```python
from build123d import *

# Parameters (mm, degrees)
SKETCH1_R           = 11
BOSS_EXTRUDE2_DEPTH = 8
SKETCH3_R           = 3
SKETCH3_R_2         = 1.5
CUT_EXTRUDE2_DEPTH  = 12
CUT_EXTRUDE3_START  = -4
SKETCH4_R           = 11
SKETCH4_R_2         = 4.5
CUT_EXTRUDE3_DEPTH  = 4
SKETCH6_R           = 3.5
CUT_EXTRUDE4_DEPTH  = 10


with BuildPart() as part:
    # Sketch1 → Boss-Extrude2 (new body)
    with BuildSketch(Plane(origin=(0, 0, 0), x_dir=(1, 0, 0), z_dir=(0, 1, 0))):
        with Locations(Location((0, 0, 0), (0, 0, 270))):
            Circle(SKETCH1_R)
    extrude(amount=BOSS_EXTRUDE2_DEPTH)

    # Sketch3 → Cut-Extrude2 (cut)
    with BuildSketch(Plane(origin=(0, 8, 0), x_dir=(1, 0, 0), z_dir=(0, 1, 0))):
        with Locations(Location((0, 0, 0), (0, 0, 270))):
            Circle(SKETCH3_R)
        with Locations(Location((-7, 0, 0), (0, 0, 270))):
            Circle(SKETCH3_R_2)
        with Locations(Location((0, 7, 0), (0, 0, 270))):
            Circle(SKETCH3_R_2)
        with Locations(Location((7, 0, 0), (0, 0, 270))):
            Circle(SKETCH3_R_2)
        with Locations(Location((0, -7, 0), (0, 0, 270))):
            Circle(SKETCH3_R_2)
    extrude(amount=-CUT_EXTRUDE2_DEPTH, mode=Mode.SUBTRACT)

    # Sketch4 → Cut-Extrude3 (cut)
    with BuildSketch(Plane(origin=(0, 8, 0), x_dir=(1, 0, 0), z_dir=(0, 1, 0)).offset(CUT_EXTRUDE3_START)):
        with Locations(Location((0, 0, 0), (0, 0, 270))):
            Circle(SKETCH4_R)
        with Locations(Location((0, 0, 0), (0, 0, 270))):
            Circle(SKETCH4_R_2, mode=Mode.SUBTRACT)
    extrude(amount=CUT_EXTRUDE3_DEPTH, mode=Mode.SUBTRACT)

    # Sketch6 → Cut-Extrude4 (cut)
    with BuildSketch(Plane(origin=(0, 8, 0), x_dir=(1, 0, 0), z_dir=(0, 1, 0))):
        with Locations(Location((0, 0, 0), (0, 0, 270))):
            Circle(SKETCH6_R)
    extrude(amount=-CUT_EXTRUDE4_DEPTH, mode=Mode.SUBTRACT)


solid = part.part
```
Source: CAD feature listing. Evaluate the final solid. Frame: model axes, mm. A direction names the side the tool comes from. Give positions to 0.01 mm unless a question says otherwise; leave off trailing zeros. Loops run counter-clockwise (first coordinate to the right, second up) from the corner with the lowest first, then second, coordinate; pieces in that order, holes last. Notation, with made-up numbers: (-35.5, 64) - (9.5, 64) arc R23 cw to (9.5, 101) - close; hole circle Ø1 at (-3, 25.25). An arc over 180 degrees is marked (long way). Use CSV: the item, a comma, the result in double quotes. Start each with the question number.
1. Section C-C (x = 2.25). Output: boundary loops of the cut face in (y, z).
2. Pin query (flat end, axial travel): pin 1 (2.5 mm diameter, centred on x = -7, z = 0, fed in from +Y); pin 2 (3 mm diameter, centred on y = 6, z = -5, fed in from -X); pin 3 (3 mm diameter, centred on y = 1, z = -7, fed in from -X); pin 4 (4 mm diameter, centred on x = 0, z = 7, fed in from +Y). Return the tip coordinate at first contact, or that it passes through.
3. Ray query, L1, parallel to X at y = 2.8, z = 0; L2, parallel to Z at x = 0.5, y = 1.75; L3, parallel to Y at x = -6, z = -6.5. Return the intervals inside material, ascending.
4. Reachability of faces 4 (the flat face through (-5, 4, 0)), 5 (the cylindrical face through (0.07, 2.03, -8.5)) from +Z, -Z, +X, -X, +Y, -Y: full face, straight path, thin tool, end or side. Return the list, or none.
5. Section A-A (z = 0). Output: boundary loops of the cut face in (x, y), then the cut area to 3 significant figures.
6. Draft query along X for faces 1 (the flat face through (-4, 8, 0)), 2 (the cylindrical face through (5.536, 2.028, -0.325)), 3 (the cylindrical face through (1.352, 5.972, 4.292)). Return one class per face: +X half, -X half, draft (parallel to the pull), parting line (faces both ways), or undercut.
7. Section D-D (z = -6). Output: boundary loops of the cut face in (x, y).
8. Section B-B (y = 1). Output: boundary loops of the cut face in (x, z).
Response:
1,outline,"(0, -10.77) - (4, -10.77) - (4, -3.9) - (8, -3.9) - (8, -2.68) - (0, -2.68) - close; (0, 2.68) - (8, 2.68) - (8, 3.9) - (4, 3.9) - (4, 10.77) - (0, 10.77) - close"
2,pin 1,"through"
2,pin 2,"x = -2.83"
2,pin 3,"x = -9.53"
2,pin 4,"y = 4"
3,L1,"-11 to -8.5, -5.5 to -3.5, 3.5 to 5.5, 8.5 to 11"
3,L2,"-10.99 to -8.41, -5.59 to -3.46, 3.46 to 5.59, 8.41 to 10.99"
3,L3,"0 to 4"
4,face 4,"+Y"
4,face 5,"+Y, -Y"
5,outline,"(-11, 0) - (-8.5, 0) - (-8.5, 4) - (-11, 4) - close; (-5.5, 0) - (-3.5, 0) - (-3.5, 8) - (-4.5, 8) - (-4.5, 4) - (-5.5, 4) - close; (3.5, 0) - (5.5, 0) - (5.5, 4) - (4.5, 4) - (4.5, 8) - (3.5, 8) - close; (8.5, 0) - (11, 0) - (11, 4) - (8.5, 4) - close"
5,area,"44.0 mm²"
6,face 1,"draft"
6,face 2,"undercut"
6,face 3,"parting line"
7,outline,"(-9.22, 0) - (-1.12, 0) - (-1.12, 4) - (-9.22, 4) - close; (1.12, 0) - (9.22, 0) - (9.22, 4) - (1.12, 4) - close"
8,outline,"circle Ø22 at (0, 0); hole circle Ø3 at (-7, 0); hole circle Ø7 at (0, 0); hole circle Ø3 at (0, -7); hole circle Ø3 at (0, 7); hole circle Ø3 at (7, 0)"
